Could you check a few things on this model? Use its own coordinates, in mm. Face numbers are marked on the shaded views. A direction names the side the tool comes from. Round coordinates to 2 decimals unless told otherwise and drop trailing zeros. Loops run counter-clockwise (first coordinate to the right, second up) from the corner with the lowest first, then second, coordinate; pieces in that order, holes last. Notation, with made-up numbers: M 11.5,57 L 33.5,57 A24 ccw 33.5,73 Z; hole C 22.5,50.5 d9. An arc over 180 degrees is marked long. One line per item, written item: value. Start each with the question number.
Q1. I'm going to push flat-ended pins straight in: pin 1 Ø8 at (x, y) = (53, -25.5) entering from +Z; pin 2 Ø14 at (y, z) = (-59.5, -45.5) entering from +X; pin 3 Ø10 at (y, z) = (-39.5, -28) entering from +X. Where does each tip first touch, or does it pass through?
Q2. Imagine slicing it at B-B (x = 56.5). Please give me the cut outline in (y, z).
Q3. Which directions (+Z, -Z, +X, -X, +Y, -Y) give clear straight access to the entire face, cutting with the end or side of a thin tool? Please do the marked faces 1, 2 and 3.
Q4. Imagine slicing it at A-A (z = -16.5). Please give me the cut outline in (x, y).
Q5. Please list where these lines run through material, in increasing order: line 1 along Z through (x, y) = (32, -20); line 2 along Y through (x, z) = (45, -38); line 3 along X through (y, z) = (-41, -9.5).
from build123d import *

# Parameters (mm, degrees)
F0_W     = 12.7
F0_H     = 50.8
F1_DEPTH = 63.5
F2_W     = 12.7
F2_H     = 50.8
F3_DEPTH = 50.8
F4_W     = 50.8
F4_H     = 12.7
F5_DEPTH = 50.8
F6_W     = 12.7
F6_H     = 12.7
F7_DEPTH = 12.7


with BuildPart() as f1:
    # F0 (on Front) → F1 (new body)
    with BuildSketch(Plane.XZ):
        with Locations((6.35, -25.4)):
            Rectangle(F0_W, F0_H)
    extrude(amount=F1_DEPTH)

    # F2 (on face) → F3 (join)
    with BuildSketch(Plane.YZ.offset(12.7)):
        with Locations((-6.35, -25.4)):
            Rectangle(F2_W, F2_H)
    extrude(amount=F3_DEPTH)

    # F4 (on face) → F5 (join)
    with BuildSketch(Plane.YZ.offset(12.7)):
        with Locations((-38.1, -44.45)):
            Rectangle(F4_W, F4_H)
    extrude(amount=F5_DEPTH)

    # F6 (on face) → F7 (cut)
    with BuildSketch(Plane.XZ.offset(63.5)):
        with Locations((57.15, -44.45)):
            Rectangle(F6_W, F6_H)
    extrude(amount=-F7_DEPTH, mode=Mode.SUBTRACT)


solid = f1.part
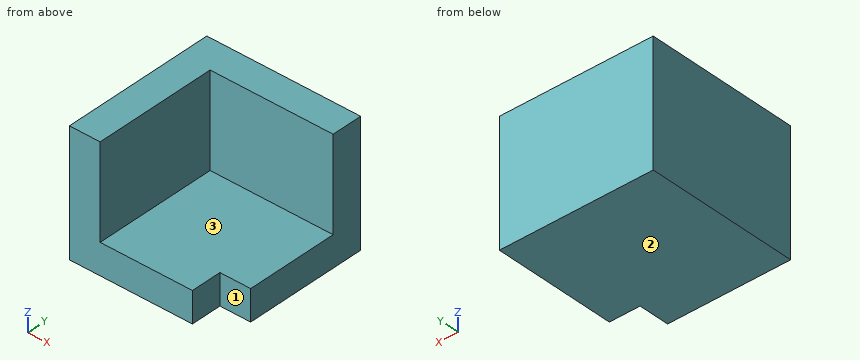
Report:
1. pin 1: stops at z = -38.1
1. pin 2: stops at x = 50.8
1. pin 3: stops at x = 12.7
2. outline: M -50.8,-50.8 L 0,-50.8 L 0,0 L -12.7,0 L -12.7,-38.1 L -50.8,-38.1 Z
3. face 1: +Z, -Z, +X, -Y
3. face 2: -Z, +X, -X, +Y, -Y
3. face 3: +Z, +X, -Y
4. outline: M 0,-63.5 L 12.7,-63.5 L 12.7,-12.7 L 63.5,-12.7 L 63.5,0 L 0,0 Z
5. line 1: z = -50.8 to -38.1
5. line 2: y = -12.7 to 0
5. line 3: x = 0 to 12.7
